Work out the finished part from the listing and answer in its coordinate system (mm). Face numbers are marked on the shaded views. Round coordinates to 2 decimals unless told otherwise and drop trailing zeros. Loops run counter-clockwise (first coordinate to the right, second up) from the corner with the lowest first, then second, coordinate; pieces in that order, holes last.
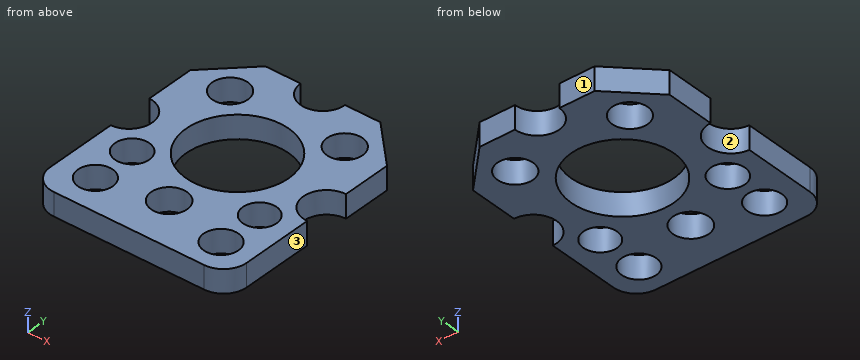
```python
from build123d import *

# Parameters (mm, degrees)
SKETCH1_W           = 21.59
SKETCH1_H           = 25.4
BOSS_EXTRUDE1_DEPTH = 2.54
FILLET1_R           = 2.54
CUT_EXTRUDE1_DEPTH  = 30.115049214
SKETCH3_R           = 5.625489831
SKETCH3_R_2         = 2.54
SKETCH3_R_3         = 2.540453657
SKETCH3_R_4         = 1.951297309
SKETCH3_R_5         = 2.434341389
SKETCH3_R_6         = 1.968933299
SKETCH3_R_7         = 1.905
CUT_EXTRUDE2_DEPTH  = 30.115049214
SKETCH4_R           = 1.851487323
SKETCH4_R_2         = 1.882954115
CUT_EXTRUDE3_DEPTH  = 30.115049214


with BuildPart() as part:
    # Sketch1 → Boss-Extrude1 (new body)
    with BuildSketch(Plane.XY):
        with Locations((-12.398804361, 4.71499153)):
            Rectangle(SKETCH1_W, SKETCH1_H)
    extrude(amount=BOSS_EXTRUDE1_DEPTH)

    # Fillet1
    fillet1_edges = [part.edges().sort_by_distance(p)[0] for p in [
        (-23.193804361, -7.98500847, 1.27),
        (-1.603804361, -7.98500847, 1.27),
    ]]
    fillet(fillet1_edges, radius=FILLET1_R)

    # Sketch2 → Cut-Extrude1 (cut, through all)
    with BuildSketch(Plane.XY.offset(2.54)):
        Polygon((-24.267164586, 11.861079729), (-17.410801404, 18.717442911), (-24.267164586, 18.717442911), align=None)
        Polygon((-7.386807318, 18.717442911), (-0.530444135, 18.717442911), (-0.530444135, 11.861079729), align=None)
    extrude(amount=-CUT_EXTRUDE1_DEPTH, mode=Mode.SUBTRACT)

    # Sketch3 → Cut-Extrude2 (cut, through all)
    with BuildSketch(Plane.XY.offset(2.54)):
        with Locations((-12.398804361, 6.226040262)):
            Circle(SKETCH3_R)
        with Locations((-23.301730566, 5.040576616)):
            Circle(SKETCH3_R_2)
        with Locations((-1.603804361, 5.023879945)):
            Circle(SKETCH3_R_3)
        with Locations((-18.693449352, 12.771135319)):
            Circle(SKETCH3_R_4)
        with Locations((-12.398804361, 17.41499153)):
            Circle(SKETCH3_R_5)
        with Locations(Location((-6.104159369, 12.771135319, 0), (0, 0, 180))):
            Circle(SKETCH3_R_4)
        with Locations((-12.398804361, -2.723375429)):
            Circle(SKETCH3_R_6)
        with Locations((-19.27783284, -4.174711925)):
            Circle(SKETCH3_R_7)
        with Locations((-5.202539132, -4.508645347)):
            Circle(SKETCH3_R_7)
    extrude(amount=-CUT_EXTRUDE2_DEPTH, mode=Mode.SUBTRACT)

    # Sketch4 → Cut-Extrude3 (cut, through all)
    with BuildSketch(Plane.XY.offset(2.54)):
        with Locations((-5.209017976, 0.565757183)):
            Circle(SKETCH4_R)
        with Locations((-19.377050407, 0.75613176)):
            Circle(SKETCH4_R_2)
    extrude(amount=-CUT_EXTRUDE3_DEPTH, mode=Mode.SUBTRACT)


solid = part.part
```
1. Find section A-A (x = -19). Write down the section's boundary in (y, z) (3 decimals).
Answer key:
outline: (-7.985, 0) - (-6.059, 0) - (-6.059, 2.54) - (-7.985, 2.54) - close; (-2.29, 0) - (-1.089, 0) - (-1.089, 2.54) - (-2.29, 2.54) - close; (2.601, 0) - (10.844, 0) - (10.844, 2.54) - (2.601, 2.54) - close; (14.698, 0) - (17.128, 0) - (17.128, 2.54) - (14.698, 2.54) - close
2. Find section C-C (z = 0.85). Give the number of separate pieces and of enclosed holes in the cut face, then the cut area to 3 significant figures.
Answer key:
separate pieces: 1
enclosed holes: 8
area: 316 mm2
3. Find section D-D (x = -14). Write down the section's boundary in (y, z) (3 decimals), then the cut area to 3 significant figures.
Answer key:
outline: (-7.985, 0) - (-3.869, 0) - (-3.869, 2.54) - (-7.985, 2.54) - close; (-1.578, 0) - (0.833, 0) - (0.833, 2.54) - (-1.578, 2.54) - close; (11.619, 0) - (15.581, 0) - (15.581, 2.54) - (11.619, 2.54) - close
area: 26.6 mm2
4. Find section B-B (y = 5). Write down the section's boundary in (x, z).
Answer key:
outline: (-20.76, 0) - (-17.89, 0) - (-17.89, 2.54) - (-20.76, 2.54) - close; (-6.91, 0) - (-4.14, 0) - (-4.14, 2.54) - (-6.91, 2.54) - close
5. Determine the mould class of the marked faces 1, 2 and 3 for opening direction Y: +Y half, -Y half, draft (parallel to the pull), parting line (faces both ways), or undercut.
Answer key:
face 1: +Y half
face 2: undercut
face 3: draft
6. Given pin 1 (4.5 mm diameter, centred on x = -19.38, y = 0.76, fed in from +Z), flat-ended and moving along its own axis, determine where the tip first touches the part or whether it passes through.
Answer key:
pin 1: stops at z = 2.54
7. Consider probe 1 along Y at (x, z) = (-13.5, 2) (3 decimals); probe 2 along X at (y, z) = (13.75, 1.6); probe 3 along X at (y, z) = (14.5, 2.2). Determine where each line is inside the solid, lowest interval first.
Answer key:
probe 1: y = -7.985 to -4.356, -1.091 to 0.709, 11.743 to 15.244
probe 2: x = -22.38 to -20.38, -17.01 to -7.79, -4.42 to -2.42
probe 3: x = -21.63 to -19.6, -17.79 to -7.01, -5.2 to -3.17
